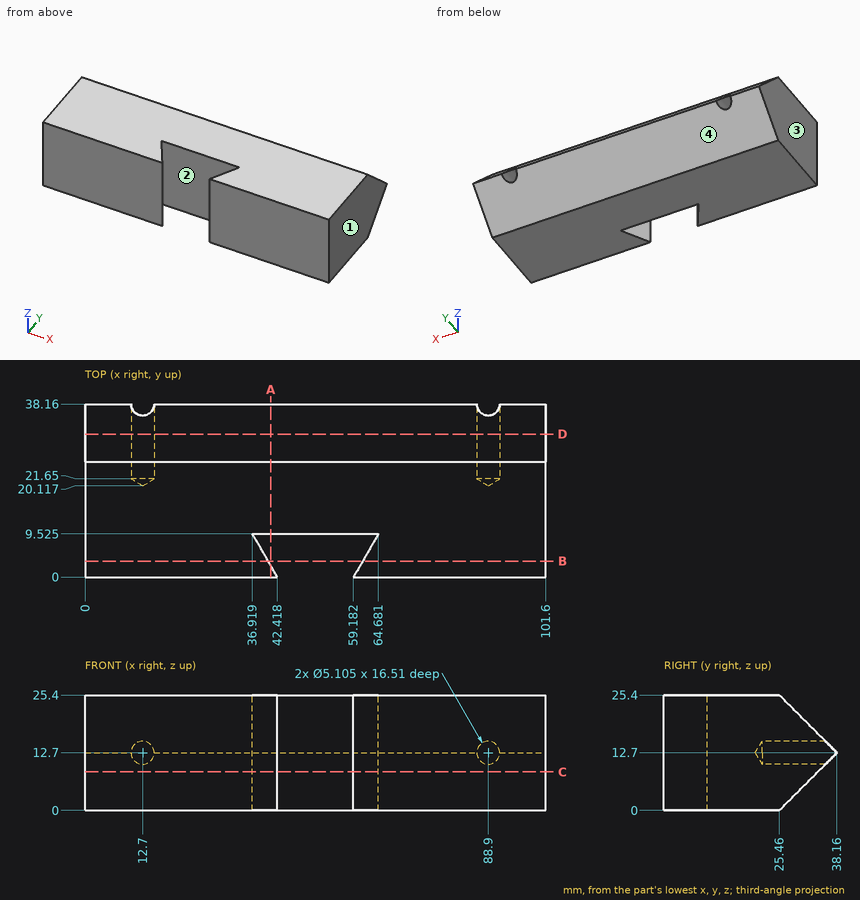
Can you work these out from the drawing? Everything is in mm from the part's minimum corner. Coordinates: 2 decimals unless noted, no trailing zeros. Loops run counter-clockwise (first coordinate to the right, second up) from the corner with the lowest first, then second, coordinate; pieces in that order, holes last. Notation, with made-up numbers: (59, -1) - (81, -1) arc R23 ccw to (81, 32) - close; hole circle Ø6 at (16, 70.5). An arc over 180 degrees is marked (long way). Use a Markdown table: item, result.
Item 1: I want a section at D-D on y = 31.5. Please give me the cut outline in (x, z) (1 decimal), and give its area (3 significant figures).
Numbers:
| item | result |
|---|---|
| outline | (0, 6) - (101.6, 6) - (101.6, 19.4) - (0, 19.4) - close; hole circle Ø5.1 at (12.7, 12.7); hole circle Ø5.1 at (88.9, 12.7) |
| area | 1,310 mm2 |
Item 2: I want a section at B-B on y = 3.5. Please give me the cut outline in (x, z), and give its area (3 significant figures).
Numbers:
| item | result |
|---|---|
| outline | (0, 0) - (40.4, 0) - (40.4, 25.4) - (0, 25.4) - close; (61.2, 0) - (101.6, 0) - (101.6, 25.4) - (61.2, 25.4) - close |
| area | 2,050 mm2 |
Item 3: I want a section at A-A on x = 41. Please give me the cut outline in (y, z) (1 decimal).
Numbers:
| item | result |
|---|---|
| outline | (0, 0) - (2.5, 0) - (2.5, 25.4) - (0, 25.4) - close; (9.5, 0) - (25.5, 0) - (38.2, 12.7) - (25.5, 25.4) - (9.5, 25.4) - close |
Item 4: Will these pins go through, and if not, where does the flat tip stop? pin 1 (6 mm diameter, centred on x = 74, y = 31, fed in from +Z); pin 2 (4 mm diameter, centred on x = 84.5, z = 21.5, fed in from +Y); pin 3 (4 mm diameter, centred on x = 88.9, z = 12.7, fed in from +Y).
Numbers:
| item | result |
|---|---|
| pin 1 | stops at z = 22.86 |
| pin 2 | stops at y = 31.36 |
| pin 3 | stops at y = 21.32 |
Item 5: If I drill on probe 1 along X at (y, z) = (34, 12.7); probe 2 along Z at (x, y) = (12.7, 25.25); probe 3 along Z at (x, y) = (15, 31) (1 decimal), over which ranges is the centre line in solid material (lowest first)? Write a range as from..to.
Numbers:
| item | result |
|---|---|
| probe 1 | x = 0..10.15, 15.25..86.35, 91.45..101.6 |
| probe 2 | z = 0..10.15, 15.25..25.4 |
| probe 3 | z = 5.5..11.6, 13.8..19.9 |
Item 6: We'd pull the mould along X, two halves only. Please class the marked faces 1, 2, 3 and 4: released by +X, released by -X, zero draft, split by the parting line, or undercut.
Numbers:
| item | result |
|---|---|
| face 1 | released by +X |
| face 2 | undercut |
| face 3 | released by -X |
| face 4 | zero draft |
Item 7: I want a section at C-C on z = 8.5. Please give me the cut outline in (x, y) (1 decimal).
Numbers:
| item | result |
|---|---|
| outline | (0, 0) - (42.4, 0) - (36.9, 9.5) - (64.7, 9.5) - (59.2, 0) - (101.6, 0) - (101.6, 34) - (0, 34) - close |
